from build123d import *

# Parameters (mm, degrees)
SKETCH1_W           = 150
SKETCH1_H           = 35
BOSS_EXTRUDE1_DEPTH = 10
SKETCH2_R           = 11.3
CUT_EXTRUDE1_DEPTH  = 8
CUT_EXTRUDE2_DEPTH  = 78.661122835
FILLET1_R           = 5
FILLET2_R           = 1


with BuildPart() as part:
    # Sketch1 → Boss-Extrude1 (new body)
    with BuildSketch(Plane.XY):
        Rectangle(SKETCH1_W, SKETCH1_H)
    extrude(amount=BOSS_EXTRUDE1_DEPTH)

    # Sketch2 → Cut-Extrude1 (cut)
    with BuildSketch(Plane.XY.offset(10)):
        with Locations((-60, 0)):
            Circle(SKETCH2_R)
        with Locations((60, 0)):
            Circle(SKETCH2_R)
    extrude(amount=-CUT_EXTRUDE1_DEPTH, mode=Mode.SUBTRACT)

    # Sketch3 → Cut-Extrude2 (cut, through all)
    with BuildSketch(Plane.XY.offset(10)):
        with BuildLine():
            Line((24.729241078, -4.501356784), (-24.729241078, -4.501356784))
            ThreePointArc((-24.729241078, -4.501356784), (-26.520071482, -4.663017165), (-28.253000621, -5.142771491))
            ThreePointArc((-28.253000621, -5.142771491), (-39.611340556, -10.468134508), (-50, -17.5))
            Line((-50, -17.5), (50, -17.5))
            ThreePointArc((50, -17.5), (39.611340556, -10.468134508), (28.253000621, -5.142771491))
            ThreePointArc((28.253000621, -5.142771491), (26.520071482, -4.663017165), (24.729241078, -4.501356784))
        make_face()
        with BuildLine():
            ThreePointArc((-28.253000621, 5.142771491), (-26.520071482, 4.663017165), (-24.729241078, 4.501356784))
            Line((-24.729241078, 4.501356784), (24.729241078, 4.501356784))
            ThreePointArc((24.729241078, 4.501356784), (26.520071482, 4.663017165), (28.253000621, 5.142771491))
            ThreePointArc((28.253000621, 5.142771491), (39.611340556, 10.468134508), (50, 17.5))
            Line((50, 17.5), (-50, 17.5))
            ThreePointArc((-50, 17.5), (-39.611340556, 10.468134508), (-28.253000621, 5.142771491))
        make_face()
    extrude(amount=-CUT_EXTRUDE2_DEPTH, mode=Mode.SUBTRACT)

    # Fillet1
    fillet1_edges = [part.edges().sort_by_distance(p)[0] for p in [
        (50, -17.5, 5),
        (-50, -17.5, 5),
        (-50, 17.5, 5),
        (50, 17.5, 5),
        (-75, 17.5, 5),
        (75, 17.5, 5),
        (75, -17.5, 5),
        (-75, -17.5, 5),
    ]]
    fillet(fillet1_edges, radius=FILLET1_R)

    # Fillet2
    fillet2_edges = [part.edges().sort_by_distance(p)[0] for p in [
        (-71.3, 0, 10),
        (48.7, 0, 10),
    ]]
    fillet(fillet2_edges, radius=FILLET2_R)


solid = part.part
Geometry: final body of the model. Coordinates: model frame, mm. A direction names the side the tool comes from. Coordinates: 2 decimals unless noted, no trailing zeros. Order: outer loops, then holes, each group sorted by start corner. A loop starts at its lowest first (then second) coordinate and runs counter-clockwise, first axis right, second up.
(1) Section query D-D (x = 23). Return the cut outline in (y, z).
(2) Material intervals for probe 1 along X at (y, z) = (-0.5, 9); probe 2 along Y at (x, z) = (-60, 4); probe 3 along X at (y, z) = (-3, 6.25), sorted ascending.
(3) First-contact query: pin 1 (7 mm diameter, centred on x = -56.5, y = -5.5, fed in from +Z); pin 2 (2 mm diameter, centred on x = -41, z = 4.5, fed in from -Y); pin 3 (1.5 mm diameter, centred on x = -17, z = 3, fed in from +Y). Flat tips, straight axial feed; report the tip coordinate or a pass-through.
(4) Section query B-B (y = 0). Return the cut outline in (x, z).
(5) Section query C-C (x = -60). Return the cut outline in (y, z).
(6) Draft query along X for faces 1 (the face through (-75, 0, 5)), 2 (the face through (39.03, -10.14, 5.07)), 3 (the face through (73.5, 16.07, 5.07)). Return one class per face: pulls with the +X half, pulls with the -X half, needs draft (parallel to the pull), parting line crosses it, or undercut.
(7) Section query A-A (z = 4.5). Return the cut outline in (x, y), plus the area to 3 significant figures.
(8) Access query for faces 4 (the face through (-50.14, -17.243, 4.93)), 5 (the face through (0, 4.501, 5)), 6 (the face through (60, 0, 2)), 7 (the face through (-61, -17.5, 5)). Directions: +Z, -Z, +X, -X, +Y, -Y. A direction counts if a zero-diameter tool reaches every point of the face in a straight line with its end or side. Return the directions, or none.
Solution:
1. outline: (-4.5, 0) - (4.5, 0) - (4.5, 10) - (-4.5, 10) - close
2. probe 1: x = -75 to -71.29, -48.71 to 48.71, 71.29 to 75
2. probe 2: y = -17.5 to -11.3, 11.3 to 17.5
2. probe 3: x = -75 to -70.89, -49.11 to 49.11, 70.89 to 75
3. pin 1: stops at z = 2
3. pin 2: stops at y = -11.88
3. pin 3: stops at y = 4.5
4. outline: (-75, 0) - (75, 0) - (75, 10) - (72.3, 10) arc R1 ccw to (71.3, 9) - (71.3, 2) - (48.7, 2) - (48.7, 9) arc R1 ccw to (47.7, 10) - (-47.7, 10) arc R1 ccw to (-48.7, 9) - (-48.7, 2) - (-71.3, 2) - (-71.3, 9) arc R1 ccw to (-72.3, 10) - (-75, 10) - close
5. outline: (-17.5, 0) - (17.5, 0) - (17.5, 10) - (12.3, 10) arc R1 ccw to (11.3, 9) - (11.3, 2) - (-11.3, 2) - (-11.3, 9) arc R1 ccw to (-12.3, 10) - (-17.5, 10) - close
6. face 1: pulls with the -X half
6. face 2: undercut
6. face 3: pulls with the +X half
7. outline: (-75, -12.5) arc R5 ccw to (-70, -17.5) - (-51.72, -17.5) arc R5 ccw to (-48.68, -16.47) arc R80.18 cw to (-28.25, -5.14) arc R10 cw to (-24.73, -4.5) - (24.73, -4.5) arc R10 cw to (28.25, -5.14) arc R80.18 cw to (48.68, -16.47) arc R5 ccw to (51.72, -17.5) - (70, -17.5) arc R5 ccw to (75, -12.5) - (75, 12.5) arc R5 ccw to (70, 17.5) - (51.72, 17.5) arc R5 ccw to (48.68, 16.47) arc R80.18 cw to (28.25, 5.14) arc R10 cw to (24.73, 4.5) - (-24.73, 4.5) arc R10 cw to (-28.25, 5.14) arc R80.18 cw to (-48.68, 16.47) arc R5 ccw to (-51.72, 17.5) - (-70, 17.5) arc R5 ccw to (-75, 12.5) - close; hole circle Ø22.6 at (-60, 0); hole circle Ø22.6 at (60, 0)
7. area: 2,360 mm2
8. face 4: +Z, -Z, -Y
8. face 5: +Z, -Z, +Y
8. face 6: +Z
8. face 7: +Z, -Z, +X, -X, -Y
